Solid Edge part; units mm, degrees
sketch "Sketch1" plane through (0, 0, -5.0832) normal (0, 0, 1) x (1, 0, 0)
  circle A0 centre (219.5, -4.0267) radius 1.7
  circle A1 centre (219.5, -11.0267) radius 1.7
  circle A2 centre (90.5, -4.0267) radius 1.7
  circle A3 centre (90.5, -11.0267) radius 1.7
  circle A4 centre (90.5, -166.0267) radius 1.7
  circle A5 centre (90.5, -159.0267) radius 1.7
  circle A6 centre (219.5, -166.0267) radius 1.7
  circle A7 centre (219.5, -159.0267) radius 1.7
  line L0 (84, -0.0267) -> (226, -0.0267)
  line L1 (226, -0.0267) -> (226, -170.0267)
  line L2 (226, -170.0267) -> (84, -170.0267)
  line L3 (84, -170.0267) -> (84, -0.0267)
  dimension "D1" = 84
  dimension "D2" = 84
extrude "ExtrudedProtrusion_1" add sketch "Sketch1" along normal blind 4.5
sketch "Sketch2" plane through (-67, -90, -0.5832) normal (0, 0, 1) x (0, -1, 0)
  circle A0 centre (-5.9733, 261) radius 1.7
  circle A1 centre (9.0267, 277) radius 1.7
  circle A2 centre (9.0267, 212) radius 1.7
  circle A3 centre (-83.9733, 167) radius 1.7
  circle A4 centre (74.0267, 277) radius 1.7
extrude "Cutout1" cut sketch "Sketch2" against normal through all
properties material "Steel"
Build history of the part. All positions in model axes, mm. Round coordinates to 2 decimals unless told otherwise and drop trailing zeros. One line per item, written item: value. Start each with the question number.
Q1. Probe line 1 along Y through (x, z) = (219.5, -2.5); line 2 along Y through (x, z) = (145, -3.25); line 3 along Y through (x, z) = (100, -4). List the from-to ranges inside material, lowest first.
Q2. Drop a flat-ended pin along its axis: pin 1 Ø2 at (x, y) = (219.5, -11.03) entering from +Z. Give the stop position or say it passes through.
Q3. Two-plate mould, pull along Y, no slides. Class faces 1 (the face through (156, -170.027, -3)), 2 (the face through (90.131, -164.367, -2.865)), 3 (the face through (156, -84, -5.083)): released by +Y, released by -Y, zero draft, split by the parting line, or undercut.
Computed:
1. line 1: -170.03 to -167.73, -164.33 to -160.73, -157.33 to -12.73, -9.33 to -5.73, -2.33 to -0.03
1. line 2: -170.03 to -100.73, -97.33 to -0.03
1. line 3: -170.03 to -7.73, -4.33 to -0.03
2. pin 1: through
3. face 1: released by -Y
3. face 2: undercut
3. face 3: zero draft
